Part model, mm, in its own coordinate system. Face numbers are marked on the shaded views. A direction names the side the tool comes from. Coordinates: 2 decimals unless noted, no trailing zeros. Order: outer loops, then holes, each group sorted by start corner. A loop starts at its lowest first (then second) coordinate and runs counter-clockwise, first axis right, second up.
from build123d import *
from build123d.topology import SkipClean

# Parameters (mm, degrees)
LEVER_R                       = 1
BOSS_EXTRUDE1_DEPTH           = 5.35
SKETCH1_R                     = 1.2
CUT_EXTRUDE1_DEPTH            = 32.557448
UPPERJAW_DEPTH                = 5.35
SKETCH5_W                     = 6
SKETCH5_H                     = 2
LOWERJAW_DEPTH                = 5.35
BANDCAPTURE_DEPTH             = 5
BANDCAPTURE_DEPTH_BACK        = 10
SKETCH6_W                     = 1.5
SKETCH6_H                     = 15
CUT_EXTRUDE3_DEPTH            = 34.316662
CUT_EXTRUDE3_DEPTH_BACK       = 34.316662
SKETCH7_W                     = 1.5
SKETCH7_H                     = 12
BATTERYCRADLEWIDTH_DEPTH      = 10
BATTERYCRADLEWIDTH_DEPTH_BACK = 15
CHAMFER1_SIZE                 = 2


with BuildPart() as part:
    # lever → Boss-Extrude1 (new body)
    with BuildSketch(Plane.XY):
        with BuildLine():
            Line((-0.75, -4.690416), (-0.75, -2.384848))
            ThreePointArc((-0.75, -2.384848), (-2.496435, -0.133467), (-1, 2.291288))
            Line((-1, 2.291288), (-1, 30))
            ThreePointArc((-1, 30), (0, 31), (1, 30))
            Line((1, 30), (1, 2.291288))
            ThreePointArc((1, 2.291288), (2.496435, -0.133467), (0.75, -2.384848))
            Line((0.75, -2.384848), (0.75, -4))
            ThreePointArc((0.75, -4), (0.53033, -4.53033), (0, -4.75))
            ThreePointArc((0, -4.75), (-0.376182, -4.735081), (-0.75, -4.690416))
        make_face()
        Circle(LEVER_R, mode=Mode.SUBTRACT)
    extrude(amount=BOSS_EXTRUDE1_DEPTH)

    # Sketch1 → Cut-Extrude1 (cut, through all)
    with BuildSketch(Plane.XY.offset(5.35)):
        Circle(SKETCH1_R)
    extrude(amount=-CUT_EXTRUDE1_DEPTH, mode=Mode.SUBTRACT)

    # Sketch4 → UpperJaw (add)
    with BuildSketch(Plane(origin=(0, 0, 0), x_dir=(-1, 0, 0), z_dir=(0, 0, -1))):
        with BuildLine():
            Line((0, 31), (7, 31))
            Line((7, 31), (7, 29))
            Line((7, 29), (1, 29))
            Line((1, 29), (1, 30))
            ThreePointArc((1, 30), (0.707107, 30.707107), (0, 31))
        make_face()
    extrude(amount=-UPPERJAW_DEPTH)

    # Sketch5 → LowerJaw (add, through all)
    with BuildSketch(Plane(origin=(0, 0, 0), x_dir=(-1, 0, 0), z_dir=(0, 0, -1))):
        with Locations((4, 8)):
            Rectangle(SKETCH5_W, SKETCH5_H)
    extrude(amount=-LOWERJAW_DEPTH)

    # Sketch6 → BandCapture (add, two sides: drawn at the far end of the back side and taken through both)
    with BuildSketch(Plane(origin=(0, 0, 0), x_dir=(-1, 0, 0), z_dir=(0, 0, -1)).offset(-BANDCAPTURE_DEPTH_BACK)):
        with Locations((-1.75, 19)):
            Rectangle(SKETCH6_W, SKETCH6_H)
    extrude(amount=BANDCAPTURE_DEPTH + BANDCAPTURE_DEPTH_BACK)

    # Sketch7 → Cut-Extrude3 (cut, two sides: drawn at the far end of the back side and taken through both)
    with BuildSketch(Plane(origin=(0, 0, 0), x_dir=(-1, 0, 0), z_dir=(0, 0, -1)).offset(-CUT_EXTRUDE3_DEPTH_BACK)):
        with Locations((-1.75, 19)):
            Rectangle(SKETCH7_W, SKETCH7_H)
    extrude(amount=CUT_EXTRUDE3_DEPTH + CUT_EXTRUDE3_DEPTH_BACK, mode=Mode.SUBTRACT)

    # Sketch8 → BatteryCradleWidth (add, two sides: drawn at the far end of the back side and taken through both)
    with SkipClean():  # the faces are left unmerged after this step: merging them gives an invalid solid
        with BuildSketch(Plane(origin=(0, 0, 0), x_dir=(-1, 0, 0), z_dir=(0, 0, -1)).offset(-BATTERYCRADLEWIDTH_DEPTH_BACK)):
            with BuildLine():
                Line((-1, 7), (7, 7))
                Line((7, 7), (7, 9))
                Line((7, 9), (1, 9))
                Line((1, 9), (1, 29))
                Line((1, 29), (7, 29))
                Line((7, 29), (7, 31))
                Line((7, 31), (0, 31))
                ThreePointArc((0, 31), (-0.707107, 30.707107), (-1, 30))
                Line((-1, 30), (-1, 7))
            make_face()
        extrude(amount=BATTERYCRADLEWIDTH_DEPTH + BATTERYCRADLEWIDTH_DEPTH_BACK)

    # Chamfer1
    # the kernel refuses this chamfer: 2 mm, written as the material it takes off along each edge
    with BuildSketch(Plane(origin=(2.5, 19.856634, 10), x_dir=(-0.9996219169112968, 0, 0.027495876610586487), z_dir=(0, 1, 0))) as chamfer1_piece_1_section:
        Polygon((CHAMFER1_SIZE * 0.999621916911, -CHAMFER1_SIZE * 0.0274958766106), (-CHAMFER1_SIZE * 0.0274958766106, -CHAMFER1_SIZE * 0.999621916911), (0, 0), align=None)
    chamfer1_piece_1 = extrude(amount=11.786732, mode=Mode.PRIVATE)
    chamfer1_piece_1 = split(chamfer1_piece_1, bisect_by=Plane(origin=(1, 25.75, 9.296082), z_dir=(1, 0, 0)), keep=Keep.TOP, mode=Mode.PRIVATE)
    add(chamfer1_piece_1, mode=Mode.SUBTRACT)
    with BuildSketch(Plane(origin=(2.5, 6.356634, 10), x_dir=(-0.9996219169112968, 0, 0.027495876610586487), z_dir=(0, 1, 0))) as chamfer1_piece_2_section:
        Polygon((CHAMFER1_SIZE * 0.999621916911, -CHAMFER1_SIZE * 0.0274958766106), (-CHAMFER1_SIZE * 0.0274958766106, -CHAMFER1_SIZE * 0.999621916911), (0, 0), align=None)
    chamfer1_piece_2 = extrude(amount=11.786732, mode=Mode.PRIVATE)
    chamfer1_piece_2 = split(chamfer1_piece_2, bisect_by=Plane(origin=(1, 12.25, 9.296082), z_dir=(1, 0, 0)), keep=Keep.TOP, mode=Mode.PRIVATE)
    add(chamfer1_piece_2, mode=Mode.SUBTRACT)
    with BuildSketch(Plane(origin=(2.5, 6.356634, -5), x_dir=(-0.9996219169112968, 0, -0.027495876610586487), z_dir=(0, 1, 0))) as chamfer1_piece_3_section:
        Polygon((CHAMFER1_SIZE * 0.999621916911, CHAMFER1_SIZE * 0.0274958766106), (-CHAMFER1_SIZE * 0.0274958766106, CHAMFER1_SIZE * 0.999621916911), (0, 0), align=None)
    chamfer1_piece_3 = extrude(amount=11.786732, mode=Mode.PRIVATE)
    chamfer1_piece_3 = split(chamfer1_piece_3, bisect_by=Plane(origin=(1, 12.25, -4.296082), z_dir=(1, 0, 0)), keep=Keep.TOP, mode=Mode.PRIVATE)
    add(chamfer1_piece_3, mode=Mode.SUBTRACT)
    with BuildSketch(Plane(origin=(2.5, 19.856634, -5), x_dir=(-0.9996219169112968, 0, -0.027495876610586487), z_dir=(0, 1, 0))) as chamfer1_piece_4_section:
        Polygon((CHAMFER1_SIZE * 0.999621916911, CHAMFER1_SIZE * 0.0274958766106), (-CHAMFER1_SIZE * 0.0274958766106, CHAMFER1_SIZE * 0.999621916911), (0, 0), align=None)
    chamfer1_piece_4 = extrude(amount=11.786732, mode=Mode.PRIVATE)
    chamfer1_piece_4 = split(chamfer1_piece_4, bisect_by=Plane(origin=(1, 25.75, -4.296082), z_dir=(1, 0, 0)), keep=Keep.TOP, mode=Mode.PRIVATE)
    add(chamfer1_piece_4, mode=Mode.SUBTRACT)


solid = part.part
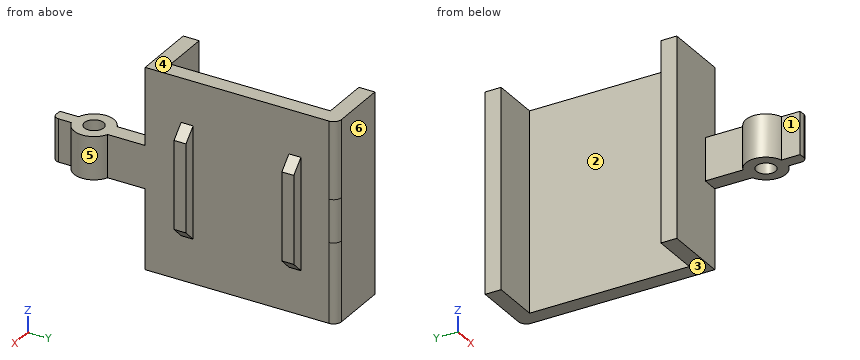
Q1. Cut at A-A on x = -5.25. Write the cut outline in (y, z).
Results list:
outline: (7, -10) - (9, -10) - (9, 15) - (7, 15) - close; (29, -10) - (31, -10) - (31, 15) - (29, 15) - close
Q2. Cut at B-B on z = 3.25. Write the cut outline in (x, y).
Results list:
outline: (-7, 7) - (-1, 7) - (-1, 2.29) arc R2.5 ccw to (-0.75, -2.38) - (-0.75, -4.69) arc R4.75 ccw to (0, -4.75) arc R0.75 ccw to (0.75, -4) - (0.75, -2.38) arc R2.5 ccw to (1, 2.29) - (1, 11.5) - (2.5, 11.5) - (2.5, 13) - (1, 13) - (1, 25) - (2.5, 25) - (2.5, 26.5) - (1, 26.5) - (1, 30) arc R1 ccw to (0, 31) - (-7, 31) - (-7, 29) - (-1, 29) - (-1, 9) - (-7, 9) - close; hole circle Ø2.4 at (0, 0)
Q3. Mould opens along Y. For the marked faces 4, 5 and 6 say: pulls with the +Y half, pulls with the -Y half, needs draft (parallel to the pull), parting line crosses it, or undercut.
Results list:
face 4: needs draft
face 5: undercut
face 6: pulls with the +Y half
Q4. Pin check, flat tips, straight feed: pin 1 Ø0.8 at (x, z) = (1.5, 1.5) entering from +Y; pin 2 Ø3 at (x, z) = (-3, 0.5) entering from -Y; pin 3 Ø4 at (x, y) = (1, 1) entering from -Z; pin 4 Ø3 at (x, y) = (-4, -1) entering from -Z. Stop position of each tip, or through.
Results list:
pin 1: stops at y = 26.5
pin 2: stops at y = -2
pin 3: stops at z = 0
pin 4: passes through
Q5. Cut at D-D on y = 0. Write the cut outline in (x, z).
Results list:
outline: (-2.5, 0) - (-1.2, 0) - (-1.2, 5.35) - (-2.5, 5.35) - close; (1.2, 0) - (2.5, 0) - (2.5, 5.35) - (1.2, 5.35) - close
Q6. Cut at C-C on x = -2. Write the cut outline in (y, z).
Results list:
outline: (-1.5, 0) - (1.5, 0) - (1.5, 5.35) - (-1.5, 5.35) - close; (7, -10) - (9, -10) - (9, 15) - (7, 15) - close; (29, -10) - (31, -10) - (31, 15) - (29, 15) - close
Q7. Which spindle directions (+Z, -Z, +X, -X, +Y, -Y) get a long thin tool onto all of the face, cutting with end or side? Do the marked faces 1, 2 and 3. Say none if no direction does.
Results list:
face 1: +Z, -Z, -X, -Y
face 2: +Z, -Z, -X
face 3: -Z, +X, -X, +Y, -Y
Q8. Wall check: line 1 along Y through (x, z) = (-5.25, 11); line 2 along Y through (x, z) = (0, 2.3); line 3 along X through (y, z) = (17, 5.25). Give the ranges that are in metal, low to high.
Results list:
line 1: y = 7 to 9, 29 to 31
line 2: y = -4.75 to -1.2, 1.2 to 31
line 3: x = -1 to 1
